Check sheet for the modelled part. Datum: model origin and axes. Units: mm. A direction names the side the tool comes from. Round coordinates to 2 decimals unless told otherwise and drop trailing zeros. Order: outer loops, then holes, each group sorted by start corner. A loop starts at its lowest first (then second) coordinate and runs counter-clockwise, first axis right, second up.
```python
from build123d import *

# Parameters (mm, degrees)
F0_W     = 69
F0_H     = 65
F1_DEPTH = 1
F2_W     = 66
F2_H     = 62
F3_DEPTH = 1
F4_R     = 1.25
F5_DEPTH = 2
F6_W     = 45.8320826292
F6_H     = 54.0132429451
F7_DEPTH = 25


with BuildPart() as f1:
    # F0 (on Top) → F1 (new body)
    with BuildSketch(Plane.XY):
        Rectangle(F0_W, F0_H)
    extrude(amount=F1_DEPTH)

    # F2 (on face) → F3 (join)
    with BuildSketch(Plane.XY.offset(1)):
        Polygon((-33, 32.5), (-34.5, 32.5), (-34.5, 31), (-34.5, -31), (-34.5, -32.5), (-33, -32.5), (33, -32.5), (34.5, -32.5), (34.5, -31), (34.5, 31), (34.5, 32.5), (33, 32.5), align=None)
        Rectangle(F2_W, F2_H, mode=Mode.SUBTRACT)
    extrude(amount=F3_DEPTH)

    # F4 (on face) → F5 (join)
    with BuildSketch(Plane.XY.offset(1)):
        with Locations((-28.6, 21.6)):
            Circle(F4_R)
        with BuildLine():
            Line((29.4, 21.6), (29.4, 20.35))
            ThreePointArc((29.4, 20.35), (30.2838834765, 20.7161165235), (30.65, 21.6))
            ThreePointArc((30.65, 21.6), (29.4, 22.85), (28.15, 21.6))
            Line((28.15, 21.6), (29.4, 21.6))
        make_face()
        with BuildLine():
            ThreePointArc((28.15, 21.6), (28.5161165235, 20.7161165235), (29.4, 20.35))
            Line((29.4, 20.35), (29.4, 21.6))
            Line((29.4, 21.6), (28.15, 21.6))
        make_face()
        with BuildLine():
            Line((28.15, -27.4), (29.4, -27.4))
            Line((29.4, -27.4), (29.4, -26.15))
            ThreePointArc((29.4, -26.15), (28.5161165235, -26.5161165235), (28.15, -27.4))
        make_face()
        with BuildLine():
            ThreePointArc((28.15, -27.4), (28.5161165235, -28.2838834765), (29.4, -28.65))
            Line((29.4, -28.65), (29.4, -27.4))
            Line((29.4, -27.4), (28.15, -27.4))
        make_face()
        with BuildLine():
            Line((29.4, -27.4), (29.4, -28.65))
            ThreePointArc((29.4, -28.65), (30.2838834765, -28.2838834765), (30.65, -27.4))
            ThreePointArc((30.65, -27.4), (30.2838834765, -26.5161165235), (29.4, -26.15))
            Line((29.4, -26.15), (29.4, -27.4))
        make_face()
        with Locations((-28.6, -27.4)):
            Circle(F4_R)
    extrude(amount=F5_DEPTH)

    # F6 (on face) → F7 (cut)
    with BuildSketch(Plane.XY.offset(1)):
        with Locations((1.0845791548, -0.7542716339)):
            Rectangle(F6_W, F6_H)
    extrude(amount=-F7_DEPTH, mode=Mode.SUBTRACT)


solid = f1.part
```
Item 1: Release check for a two-part mould opening along X. For faces 3 (the flat face through (34.5, 0, 1)), 4 (the cylindrical face through (-27.928, 22.654, 1.986)), 5 (the flat face through (-29, 22, 3)) record: released by +X, released by -X, zero draft, split by the parting line, or undercut.
Answer:
face 3: released by +X
face 4: undercut
face 5: zero draft
Item 2: Sectioned sample at D-D (x = -28.6). Record the cut outline in (y, z), and give its area (3 significant figures).
Answer:
outline: (-32.5, 0) - (32.5, 0) - (32.5, 2) - (31, 2) - (31, 1) - (22.85, 1) - (22.85, 3) - (20.35, 3) - (20.35, 1) - (-26.15, 1) - (-26.15, 3) - (-28.65, 3) - (-28.65, 1) - (-31, 1) - (-31, 2) - (-32.5, 2) - close
area: 78.0 mm2
Item 3: Sectioned sample at A-A (y = -19). Record the cut outline in (x, z), and give its area (3 significant figures).
Answer:
outline: (-34.5, 0) - (-21.83, 0) - (-21.83, 1) - (-33, 1) - (-33, 2) - (-34.5, 2) - close; (24, 0) - (34.5, 0) - (34.5, 2) - (33, 2) - (33, 1) - (24, 1) - close
area: 26.2 mm2
Item 4: Go/stop test with a flat-tipped pin: P1, Ø6, axis at x = -22, y = 10.5, coming from the -Z side. Record where the tip stops, or that it passes through.
Answer:
P1: stops at z = 0
Item 5: Sectioned sample at B-B (x = 6.5). Record the cut outline in (y, z), and give its area (3 significant figures).
Answer:
outline: (-32.5, 0) - (-27.76, 0) - (-27.76, 1) - (-31, 1) - (-31, 2) - (-32.5, 2) - close; (26.25, 0) - (32.5, 0) - (32.5, 2) - (31, 2) - (31, 1) - (26.25, 1) - close
area: 14.0 mm2
Item 6: Access from +Z, -Z, +X, -X, +Y, -Y to the whole of each face (thin tool, end or side, straight path). Record for faces 1 (the flat face through (-22, 7, 1)), 2 (the flat face through (-34.5, 0, 1)).
Answer:
face 1: +Z
face 2: +Z, -Z, -X, +Y, -Y
Item 7: Scan lines: line 1 along Y through (x, z) = (-24.5, 1.3); line 2 along X through (y, z) = (8, 1.7); line 3 along X through (y, z) = (11.5, 0.85). Record each from-to range of solid material in increasing order.
Answer:
line 1: y = -32.5 to -31, 31 to 32.5
line 2: x = -34.5 to -33, 33 to 34.5
line 3: x = -34.5 to -21.83, 24 to 34.5
Item 8: Sectioned sample at C-C (x = 26.5). Record the cut outline in (y, z), and give its area (3 significant figures).
Answer:
outline: (-32.5, 0) - (32.5, 0) - (32.5, 2) - (31, 2) - (31, 1) - (-31, 1) - (-31, 2) - (-32.5, 2) - close
area: 68.0 mm2
